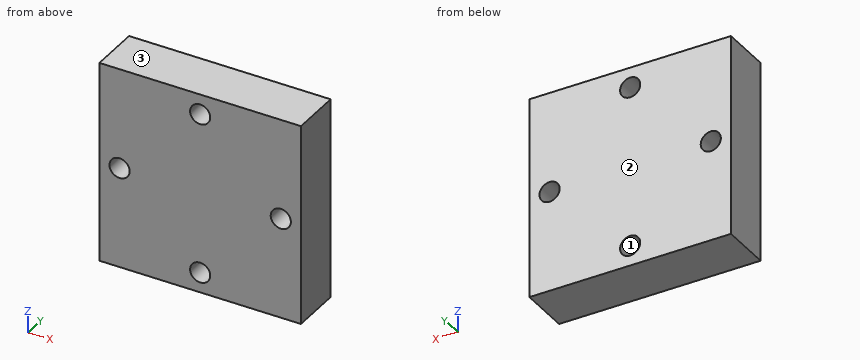
Autodesk Inventor part; units mm, degrees
ref_plane "YZ Plane" through (0, 0, 0) normal (1, 0, 0) x (0, 1, 0)
ref_plane "XZ Plane" through (0, 0, 0) normal (0, 1, 0) x (-1, 0, 0)
ref_plane "XY Plane" through (0, 0, 0) normal (0, 0, 1) x (1, 0, 0)
sketch "Sketch1" plane through (0, 0, 0) normal (0, 1, 0) x (-1, 0, 0)
  circle A0 centre (0, 0) radius 31.75
  line L0 (-31.75, -31.75) -> (31.75, -31.75)
  line L1 (31.75, -31.75) -> (31.75, 31.75)
  line L2 (31.75, 31.75) -> (-31.75, 31.75)
  line L3 (-31.75, 31.75) -> (-31.75, -31.75)
  line L4 (-31.75, -31.75) -> (31.75, 31.75) construction
  line L5 (31.75, -31.75) -> (-31.75, 31.75) construction
  point P0 (-31.75, 0)
  point P1 (0, 31.75)
  point P2 (0, -31.75)
  point P3 (31.75, 0)
  dimension "d0" = 63.5
extrude "Extrusion1" add sketch "Sketch1" along normal blind 15.875
sketch "Sketch2" plane through (0, 15.875, 0) normal (0, 1, 0) x (1, 0, 0)
  circle A0 centre (25.4, 0) radius 3.175
  circle A1 centre (0, 25.4) radius 3.175
  circle A2 centre (-25.4, 0) radius 3.175
  circle A3 centre (0, -25.4) radius 3.175
  point P0 (0, 0)
  dimension "d3" = 6.35
  dimension "d6" = 0
  dimension "d7" = 25.4
  dimension "d10" = 360
extrude "Extrusion2" cut sketch "Sketch2" against normal blind 50.8
properties part number "FrontPlatePostNoKey"
Geometry check sheet. Reference: the model listing, model coordinates, mm. Face numbers are marked on the shaded views. Round coordinates to 2 decimals unless told otherwise and drop trailing zeros. Write each loop counter-clockwise with the first axis right and the second up, starting at its lowest first coordinate (ties: lowest second). Pieces come first, ordered by that corner, then holes. Notation, with made-up numbers: (53, 55.25) - (88, 55.25) arc R17 ccw to (88, 61.25) - close; hole circle Ø8 at (-32, -39). An arc over 180 degrees is marked (long way). One line per item, written item: value.
1. Depth check by flat-ended pin: pin 1 Ø10 at (x, z) = (0, 25.4) entering from -Y; pin 2 Ø5.5 at (x, z) = (25.4, 0) entering from -Y. Enter the tip coordinate at first touch or a pass-through.
The answers:
pin 1: stops at y = 0
pin 2: passes through
2. Cross-section at A-A on z = 0. Record the boundary of the cut face in (x, y) (3 decimals), and give its area (3 significant figures).
The answers:
outline: (-31.75, 0) - (-28.575, 0) - (-28.575, 15.875) - (-31.75, 15.875) - close; (-22.225, 0) - (22.225, 0) - (22.225, 15.875) - (-22.225, 15.875) - close; (28.575, 0) - (31.75, 0) - (31.75, 15.875) - (28.575, 15.875) - close
area: 806 mm^2
3. Cross-section at D-D on x = 0. Record the boundary of the cut face in (y, z) (3 decimals), and give its area (3 significant figures).
The answers:
outline: (0, -31.75) - (15.875, -31.75) - (15.875, -28.575) - (0, -28.575) - close; (0, -22.225) - (15.875, -22.225) - (15.875, 22.225) - (0, 22.225) - close; (0, 28.575) - (15.875, 28.575) - (15.875, 31.75) - (0, 31.75) - close
area: 806 mm^2
4. Mould release check, pull along Z, two halves, no side actions. Record for the marked faces 1, 2 and 3: released by +Z, released by -Z, zero draft, split by the parting line, or undercut.
The answers:
face 1: undercut
face 2: zero draft
face 3: released by +Z
5. Cross-section at C-C on z = -25.4. Record the boundary of the cut face in (x, y) (3 decimals), and give its area (3 significant figures).
The answers:
outline: (-31.75, 0) - (-3.175, 0) - (-3.175, 15.875) - (-31.75, 15.875) - close; (3.175, 0) - (31.75, 0) - (31.75, 15.875) - (3.175, 15.875) - close
area: 907 mm^2
6. Scan lines: L1, parallel to Z at x = 0, y = 4.25 (3 decimals); L2, parallel to Z at x = -25.4, y = 3.5 (3 decimals). Record each from-to range of solid material in increasing order.
The answers:
L1: z = -31.75 to -28.575, -22.225 to 22.225, 28.575 to 31.75
L2: z = -31.75 to -3.175, 3.175 to 31.75
7. Cross-section at B-B on x = -25.4. Record the boundary of the cut face in (y, z) (3 decimals), and give its area (3 significant figures).
The answers:
outline: (0, -31.75) - (15.875, -31.75) - (15.875, -3.175) - (0, -3.175) - close; (0, 3.175) - (15.875, 3.175) - (15.875, 31.75) - (0, 31.75) - close
area: 907 mm^2
